```python
from build123d import *

# Parameters (mm, degrees)
SKETCH1_W                      = 114.3
SKETCH1_H                      = 152.4
BASE_FLANGE1_DEPTH             = 3.175
EDGE_FLANGE1_STRIP_W           = 18.700000192
EDGE_FLANGE1_STRIP_H           = 3.175
EDGE_FLANGE1_STRIP_CUT_DEPTH   = 152.4
EDGE_FLANGE1_STRIP_2_W         = 18.700000192
EDGE_FLANGE1_STRIP_2_H         = 3.175
EDGE_FLANGE1_STRIP_CUT_2_DEPTH = 152.4
EDGE_FLANGE1_DEPTH             = 152.4
EDGE_FLANGE1_BEND_DEPTH        = 152.4
FILLET1_R                      = 6.35


# Sheet-metal steps are written as plain solids
with BuildPart() as part:
    # Sketch1 → Base-Flange1 (new body)
    with BuildSketch(Plane(origin=(0, 0, 0), x_dir=(1, 0, 0), z_dir=(0, 1, 0))):
        Rectangle(SKETCH1_W, SKETCH1_H)
    extrude(amount=-BASE_FLANGE1_DEPTH)

    # Edge-Flange1 strip (across the edge) → Edge-Flange1 strip cut (cut)
    with BuildSketch(Plane(origin=(57.15, -3.175, -76.2), x_dir=(-1, 0, 0), z_dir=(0, 0, 1))):
        with Locations((-6.35, -1.5875)):
            Rectangle(EDGE_FLANGE1_STRIP_W, EDGE_FLANGE1_STRIP_H)
    extrude(amount=EDGE_FLANGE1_STRIP_CUT_DEPTH, mode=Mode.SUBTRACT)

    # Edge-Flange1 strip 2 (across the edge) → Edge-Flange1 strip cut 2 (cut)
    with BuildSketch(Plane(origin=(-57.15, -3.175, 76.2), x_dir=(1, 0, 0), z_dir=(0, 0, -1))):
        with Locations((-6.35, -1.5875)):
            Rectangle(EDGE_FLANGE1_STRIP_2_W, EDGE_FLANGE1_STRIP_2_H)
    extrude(amount=EDGE_FLANGE1_STRIP_CUT_2_DEPTH, mode=Mode.SUBTRACT)

    # Edge-Flange1 section (across the edge) → Edge-Flange1 (add)
    with BuildSketch(Plane(origin=(57.15, -3.175, -76.2), x_dir=(-1, 0, 0), z_dir=(0, 0, 1))):
        with BuildLine():
            Line((-3.175, 3.000000096), (-3.175, 73.025))
            Line((-3.175, 73.025), (0, 73.025))
            Line((0, 73.025), (0, 3.000000096))
            ThreePointArc((0, 3.000000096), (0.878679685, 0.878679685), (3.000000096, 0))
            Line((3.000000096, 0), (3.000000096, -3.175))
            ThreePointArc((3.000000096, -3.175), (-1.366384346, -1.366384346), (-3.175, 3.000000096))
        make_face()
    extrude(amount=EDGE_FLANGE1_DEPTH)

    # Edge-Flange1 section 2 (across the edge) → Edge-Flange1 bend (add)
    with BuildSketch(Plane(origin=(-57.15, -3.175, 76.2), x_dir=(1, 0, 0), z_dir=(0, 0, -1))):
        with BuildLine():
            Line((-3.175, 3.000000096), (-3.175, 73.025))
            Line((-3.175, 73.025), (0, 73.025))
            Line((0, 73.025), (0, 3.000000096))
            ThreePointArc((0, 3.000000096), (0.878679685, 0.878679685), (3.000000096, 0))
            Line((3.000000096, 0), (3.000000096, -3.175))
            ThreePointArc((3.000000096, -3.175), (-1.366384346, -1.366384346), (-3.175, 3.000000096))
        make_face()
    extrude(amount=EDGE_FLANGE1_BEND_DEPTH)

    # Fillet1
    fillet1_edges = [part.edges().sort_by_distance(p)[0] for p in [
        (58.7375, -76.2, -76.2),
        (58.7375, -76.2, 76.2),
        (-58.7375, -76.2, 76.2),
        (-58.7375, -76.2, -76.2),
    ]]
    fillet(fillet1_edges, radius=FILLET1_R)


solid = part.part
```
Input: part model. Units: mm. Frame: model coordinates. A direction names the side the tool comes from. Coordinates: 2 decimals unless noted, no trailing zeros. Order: outer loops, then holes, each group sorted by start corner. A loop starts at its lowest first (then second) coordinate and runs counter-clockwise, first axis right, second up. Notation, with made-up numbers: (20.25, -24.5) - (40.25, -24.5) arc R8 cw to (40.25, -20.5) - close; hole circle Ø3 at (84.5, 60.5). An arc over 180 degrees is marked (long way). Put each result on its own line as item: value.
1. Cut plane B-B on z = -2. Return the cut outline in (x, y) (3 decimals).
Report:
outline: (-60.325, -76.2) - (-57.15, -76.2) - (-57.15, -6.175) arc R3 cw to (-54.15, -3.175) - (54.15, -3.175) arc R3 cw to (57.15, -6.175) - (57.15, -76.2) - (60.325, -76.2) - (60.325, -6.175) arc R6.175 ccw to (54.15, 0) - (-54.15, 0) arc R6.175 ccw to (-60.325, -6.175) - close
2. Line query: line 1 along X through (y, z) = (-29.5, -12) (3 decimals); line 2 along Y through (x, z) = (-43, -18.5) (3 decimals). Output: solid intervals per line, ascending.
Report:
line 1: x = -60.325 to -57.15, 57.15 to 60.325
line 2: y = -3.175 to 0
3. Cut plane C-C on x = -25. Return the cut outline in (y, z) (3 decimals), then the cut area to 3 significant figures.
Report:
outline: (-3.175, -76.2) - (0, -76.2) - (0, 76.2) - (-3.175, 76.2) - close
area: 484 mm2
4. Reachability of faces 5 (the face through (-1, -3.175, -1)), 6 (the face through (58.47, -1.76, -1.07)) from +Z, -Z, +X, -X, +Y, -Y: full face, straight path, thin tool, end or side. Return the list, or none.
Report:
face 5: +Z, -Z, -Y
face 6: +Z, -Z, +X, +Y
5. Cut plane A-A on y = -40.5. Return the cut outline in (x, z) (3 decimals).
Report:
outline: (-60.325, -76.2) - (-57.15, -76.2) - (-57.15, 76.2) - (-60.325, 76.2) - close; (57.15, -76.2) - (60.325, -76.2) - (60.325, 76.2) - (57.15, 76.2) - close
6. Contact query for a flat-ended pin moving along its axis: pin 1 Ø8 at (x, z) = (36.5, -40) entering from -Y (3 decimals). Output: stop coordinate, or through.
Report:
pin 1: stops at y = -3.175
7. Draft query along X for faces 1 (the face through (60.325, -41, -1)), 2 (the face through (57.15, -42, -1)), 3 (the face through (-58.72, -74.39, 74.29)), 4 (the face through (-58.47, -1.76, 1.07)). Return one class per face: pulls with the +X half, pulls with the -X half, needs draft (parallel to the pull), parting line crosses it, or undercut.
Report:
face 1: pulls with the +X half
face 2: undercut
face 3: needs draft
face 4: pulls with the -X half
